Work out the finished part from the listing and answer in its coordinate system (mm). Face numbers are marked on the shaded views. A direction names the side the tool comes from. Round coordinates to 2 decimals unless told otherwise and drop trailing zeros. Order: outer loops, then holes, each group sorted by start corner. A loop starts at its lowest first (then second) coordinate and runs counter-clockwise, first axis right, second up. Notation, with made-up numbers: (50, 9.5) - (97, 9.5) arc R36 cw to (97, 48.5) - close; hole circle Ø8 at (-20, 57.5). An arc over 180 degrees is marked (long way). Use CSV: the item, a comma, the result in double quotes.
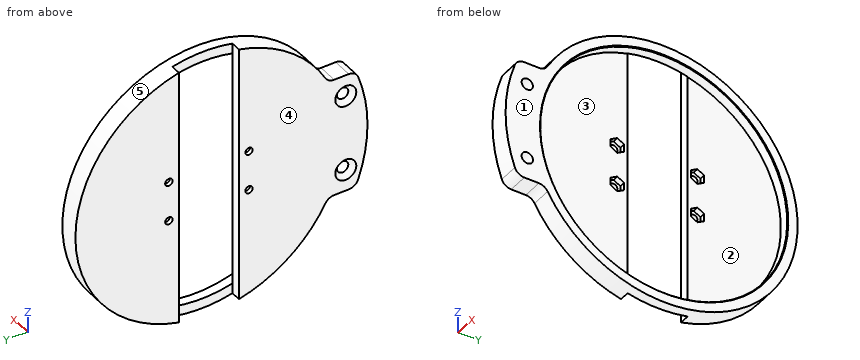
from build123d import *

# Parameters (mm, degrees)
CHAMFER_2_SIZE              = 0.2
CUT_EXTRUDE_START           = -10
CUT_EXTRUDE_1_DEPTH         = 10
HOLE_WIZARD_M31_D           = 3.4
HOLE_WIZARD_M31_CSINK_D     = 6.3
HOLE_WIZARD_M31_CSINK_ANGLE = 90
FILLET_1_R                  = 3
SKETCH_5_W                  = 80
SKETCH_5_H                  = 18
CUT_EXTRUDE_2_DEPTH         = 3
HOLE_WIZARD_M21_D           = 2.2
CUT_EXTRUDE_3_DEPTH         = 1.7


with BuildPart() as part:
    # Эскиз1 → Повернуть1 (revolve)
    with BuildSketch(Plane.XY, mode=Mode.PRIVATE) as revolve_1_sk:
        Polygon((6, 37), (2.9, 37), (2.9, 0), (0, 0), (0, 47.5), (6, 47.5), align=None)
    revolve(revolve_1_sk.sketch.rotate(Axis((-5.881924198, 0, 0), (1, 0, 0)), 90), axis=Axis((-5.881924198, 0, 0), (1, 0, 0)))

    # Фаска2
    chamfer_2_edges = [part.edges().sort_by_distance(p)[0] for p in [
        (6, 0, -37),
    ]]
    chamfer(chamfer_2_edges, length=CHAMFER_2_SIZE)

    # Эскиз2 → Вырез-Вытянуть1 (cut)
    with BuildSketch(Plane.ZY.offset(CUT_EXTRUDE_START)):
        with BuildLine():
            Line((-18, -35.721142199), (-18, -43.957365708))
            ThreePointArc((-18, -43.957365708), (0, 47.5), (18, -43.957365708))
            Line((18, -43.957365708), (18, -35.721142199))
            ThreePointArc((18, -35.721142199), (0, 40), (-18, -35.721142199))
        make_face()
    extrude(amount=CUT_EXTRUDE_1_DEPTH, mode=Mode.SUBTRACT)

    # Зенковка для винта с потайной головкой M31 (through all)
    with Locations(Plane.ZY):
        with Locations((-11.5, -41), (11.5, -41)):
            CounterSinkHole(HOLE_WIZARD_M31_D / 2, HOLE_WIZARD_M31_CSINK_D / 2, counter_sink_angle=HOLE_WIZARD_M31_CSINK_ANGLE)

    # Скругление1
    fillet_1_edges = [part.edges().sort_by_distance(p)[0] for p in [
        (3, -35.721142199, 18),
        (3, -35.721142199, -18),
        (3, -43.957365708, -18),
        (3, -43.957365708, 18),
    ]]
    fillet(fillet_1_edges, radius=FILLET_1_R)

    # Эскиз5 → Вырез-Вытянуть2 (cut)
    with BuildSketch(Plane.ZY):
        Rectangle(SKETCH_5_W, SKETCH_5_H)
    extrude(amount=-CUT_EXTRUDE_2_DEPTH, mode=Mode.SUBTRACT)

    # Отверстие с зазором M21 (through all)
    with Locations(Plane.ZY):
        with Locations((6, 12), (-6, 12), (-6, -12), (6, -12)):
            Hole(HOLE_WIZARD_M21_D / 2)

    # Эскиз8 → Вырез-Вытянуть3 (cut)
    with BuildSketch(Plane(origin=(2.9, 0, 0), x_dir=(0, 0, -1), z_dir=(1, 0, 0))):
        Polygon((7.154700538, 10), (8.309401077, 12), (7.154700538, 14), (4.845299462, 14), (3.690598923, 12), (4.845299462, 10), align=None)
        Polygon((-4.845299462, 10), (-3.690598923, 12), (-4.845299462, 14), (-7.154700538, 14), (-8.309401077, 12), (-7.154700538, 10), align=None)
        Polygon((-4.845299462, -14), (-3.690598923, -12), (-4.845299462, -10), (-7.154700538, -10), (-8.309401077, -12), (-7.154700538, -14), align=None)
        Polygon((7.154700538, -14), (8.309401077, -12), (7.154700538, -10), (4.845299462, -10), (3.690598923, -12), (4.845299462, -14), align=None)
    extrude(amount=-CUT_EXTRUDE_3_DEPTH, mode=Mode.SUBTRACT)


solid = part.part
(1) Find the intervals of material crossed by L1, parallel to Z at x = 5.5, y = -9; L2, parallel to Y at x = 0.3, z = 6; L3, parallel to Z at x = 5.05, y = -41, in increasing order. Write a range as from..to.
Findings below:
L1,"z = -38.97..-35.89, 35.89..38.97"
L2,"y = -47.12..-13.1, -10.9..-9, 9..10.9, 13.1..39.55"
L3,"z = -18..-13.2, -9.8..9.8, 13.2..18"
(2) The mould has two halves that part along Z. Classify the marked faces 3, 4 and 5: released by +Z, released by -Z, zero draft, split by the parting line, or undercut.
Findings below:
face 3,"undercut"
face 4,"zero draft"
face 5,"split by the parting line"
(3) Find section B-B (x = 4). Determine the outline of the cut face in (y, z), and give its area (3 significant figures).
Findings below:
outline,"(-44.72, -16.01) arc R3 ccw to (-41.9, -18) - (-37.52, -18) arc R3 cw to (-34.91, -19.53) arc R40 ccw (long way) to (-34.91, 19.53) arc R3 cw to (-37.52, 18) - (-41.9, 18) arc R3 ccw to (-44.72, 16.01) arc R47.5 ccw to start; hole circle Ø3.4 at (-41, -11.5); hole circle Ø3.4 at (-41, 11.5); hole circle Ø74 at (0, 0)"
area,"985 mm²"
(4) For the marked faces 1 and 2, determine the directions among +Z, -Z, +X, -X, +Y, -Y from which every point of the face is accessible in a straight line to the end or side of a thin tool.
Findings below:
face 1,"+Z, -Z, +X, +Y, -Y"
face 2,"+X"
(5) Find section A-A (z = 0). Determine the outline of the cut face in (x, y).
Findings below:
outline,"(0, -47.5) - (6, -47.5) - (6, -37.2) - (5.8, -37) - (2.9, -37) - (2.9, -9) - (0, -9) - close; (0, 9) - (2.9, 9) - (2.9, 37) - (5.8, 37) - (6, 37.2) - (6, 40) - (0, 40) - close"
(6) Find section C-C (z = -11.5). State how many separate pieces and enclosed holes the cut face has, and give its area (3 significant figures).
Findings below:
separate pieces,"3"
enclosed holes,"0"
area,"214 mm²"
(7) Each of these flat-tipped pins is pushed along its axis until it touches: pin 1 (1 mm diameter, centred on x = 2, y = -17.5, fed in from +Z); pin 2 (3 mm diameter, centred on y = 12, z = 5, fed in from +X); pin 3 (1.3 mm diameter, centred on x = 4, y = -39, fed in from -Z). Where does it stop, or does it pass through?
Findings below:
pin 1,"stops at z = 36.21"
pin 2,"stops at x = 2.9"
pin 3,"stops at z = -18"
